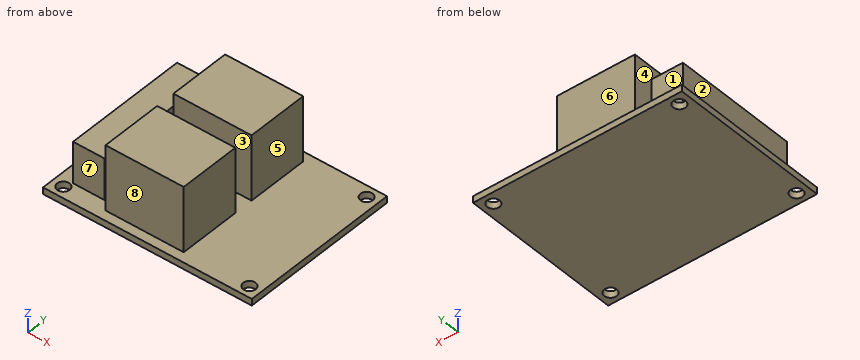
```python
from build123d import *

# Parameters (mm, degrees)
F0_W     = 50.5
F0_H     = 39
F0_R     = 1.5
F1_DEPTH = 1.6
F2_W     = 18.9
F2_H     = 14.9
F3_DEPTH = 15.7
F4_W     = 7.6
F4_H     = 30
F5_DEPTH = 10


with BuildPart() as f1:
    # F0 (on Top) → F1 (new body)
    with BuildSketch(Plane.XY):
        Rectangle(F0_W, F0_H)
        with Locations((-22.5, -16.9)):
            Circle(F0_R, mode=Mode.SUBTRACT)
        with Locations((22.5, -16.9)):
            Circle(F0_R, mode=Mode.SUBTRACT)
        with Locations((-22.5, 16.9)):
            Circle(F0_R, mode=Mode.SUBTRACT)
        with Locations((22.5, 16.9)):
            Circle(F0_R, mode=Mode.SUBTRACT)
    extrude(amount=F1_DEPTH)

    # F2 (on face) → F3 (join)
    with BuildSketch(Plane.XY.offset(1.6)):
        with Locations((-2.6, 9.822445)):
            Rectangle(F2_W, F2_H)
        with Locations((-2.6, -9.752966)):
            Rectangle(F2_W, F2_H)
    extrude(amount=F3_DEPTH)

    # F4 (on face) → F5 (join)
    with BuildSketch(Plane.XY.offset(1.6)):
        with Locations((-17.95, 0)):
            Rectangle(F4_W, F4_H)
    extrude(amount=F5_DEPTH)


solid = f1.part
```
Could you check a few things on this model? Use its own coordinates, in mm. Face numbers are marked on the shaded views. A direction names the side the tool comes from. Round coordinates to 2 decimals unless told otherwise and drop trailing zeros. Loops run counter-clockwise (first coordinate to the right, second up) from the corner with the lowest first, then second, coordinate; pieces in that order, holes last. Notation, with made-up numbers: (-15, 71.5) -> (2, 71.5) arc R12 cw to (2, 81.5) -> close; hole circle Ø8 at (36, 31). An arc over 180 degrees is marked (long way). Put each result on its own line as item: value.
Q1. I want a section at D-D on x = -1.5. Write out the boundary of the cut face in (y, z).
Checks:
outline: (-19.5, 0) -> (19.5, 0) -> (19.5, 1.6) -> (17.27, 1.6) -> (17.27, 17.3) -> (2.37, 17.3) -> (2.37, 1.6) -> (-2.3, 1.6) -> (-2.3, 17.3) -> (-17.2, 17.3) -> (-17.2, 1.6) -> (-19.5, 1.6) -> close
Q2. I want a section at A-A on z = 14.5. Write out the boundary of the cut face in (x, y).
Checks:
outline: (-12.05, -17.2) -> (6.85, -17.2) -> (6.85, -2.3) -> (-12.05, -2.3) -> close; (-12.05, 2.37) -> (6.85, 2.37) -> (6.85, 17.27) -> (-12.05, 17.27) -> close
Q3. For pin 1 Ø2.5 at (x, y) = (-22.5, -16.9) entering from -Z; pin 2 Ø8 at (x, y) = (17, -9) entering from +Z; pin 3 Ø5 at (x, y) = (-22.5, 16.9) entering from +Z; pin 4 Ø6 at (x, z) = (-16.5, 6) entering from +Y, each with a flat end and sliding along its axis, tell me the tip position at first contact or that it passes through.
Checks:
pin 1: through
pin 2: z = 1.6
pin 3: z = 11.6
pin 4: y = 15
Q4. I want a section at C-C on y = -1. Write out the boundary of the cut face in (x, z).
Checks:
outline: (-25.25, 0) -> (25.25, 0) -> (25.25, 1.6) -> (-14.15, 1.6) -> (-14.15, 11.6) -> (-21.75, 11.6) -> (-21.75, 1.6) -> (-25.25, 1.6) -> close
Q5. Thinking about a two-plate mould opening in Y: for the marked faces 1, 2 and 3, which applies, pulls with the +Y half, pulls with the -Y half, needs draft (parallel to the pull), parting line crosses it, or undercut?
Checks:
face 1: pulls with the +Y half
face 2: needs draft
face 3: undercut
Q6. Please list where these lines run through material, in increasing order: line 1 (Y direction, x = 22.5, z = 1.05); line 2 (X direction, y = 4.5, z = 6); line 3 (Y direction, x = -8.5, z = 9.25). Write a range as from..to.
Checks:
line 1: -19.5..-18.4, -15.4..15.4, 18.4..19.5
line 2: -21.75..-14.15, -12.05..6.85
line 3: -17.2..-2.3, 2.37..17.27
Q7. Which directions (+Z, -Z, +X, -X, +Y, -Y) give clear straight access to the entire face, cutting with the end or side of a thin tool? Please do the marked faces 4, 5, 6, 7 and 8.
Checks:
face 4: +Z, +Y, -Y
face 5: +Z, +X, +Y, -Y
face 6: +Z, +X, -X, +Y
face 7: +Z, -X, -Y
face 8: +Z, +X, -X, -Y
Q8. I want a section at B-B on x = -22.5. Write out the boundary of the cut face in (y, z), and give its area (3 significant figures).
Checks:
outline: (-19.5, 0) -> (-18.4, 0) -> (-18.4, 1.6) -> (-19.5, 1.6) -> close; (-15.4, 0) -> (15.4, 0) -> (15.4, 1.6) -> (-15.4, 1.6) -> close; (18.4, 0) -> (19.5, 0) -> (19.5, 1.6) -> (18.4, 1.6) -> close
area: 52.8 mm2
